Build history of the part. All positions in model axes, mm. Face numbers are marked on the shaded views. Round coordinates to 2 decimals unless told otherwise and drop trailing zeros. Loops run counter-clockwise (first coordinate to the right, second up) from the corner with the lowest first, then second, coordinate; pieces in that order, holes last. Notation, with made-up numbers: (-15, 78) - (-7, 78) arc R18 cw to (-7, 85) - close; hole circle Ø2 at (-2.75, 43.25). An arc over 180 degrees is marked (long way). Put each result on its own line as item: value. Start each with the question number.
from build123d import *

# Parameters (mm, degrees)
SKETCH051_R     = 40
PAD040_DEPTH    = 12
POCKET008_DEPTH = 12
FILLET002_R     = 1


with BuildPart() as part:
    # Sketch051 → Pad040 (new body)
    with BuildSketch(Plane.YZ.offset(67.95)):
        Circle(SKETCH051_R)
        with BuildLine():
            ThreePointArc((-1.4005, 2.125), (0, -2.545), (1.4005, 2.125))
            Line((-1.4005, 2.125), (1.4005, 2.125))
        make_face(mode=Mode.SUBTRACT)
    extrude(amount=PAD040_DEPTH)

    # Sketch052 (on Face5 of Pad040) → Pocket008 (cut)
    with BuildSketch(Plane.YZ.offset(79.95)):
        with BuildLine():
            ThreePointArc((-12.5, 31.618824), (-24.041631, 24.041631), (-31.618824, 12.5))
            ThreePointArc((-31.618824, 12.5), (-24.458371, -3.572618), (-7.720294, -8.99829))
            ThreePointArc((-12.5, 31.618824), (-22.685955, 9.830382), (-7.720294, -8.99829))
        make_face()
        with BuildLine():
            ThreePointArc((31.618824, 12.5), (24.041631, 24.041631), (12.5, 31.618824))
            ThreePointArc((12.5, 31.618824), (-3.572618, 24.458371), (-8.99829, 7.720294))
            ThreePointArc((31.618824, 12.5), (9.830382, 22.685955), (-8.99829, 7.720294))
        make_face()
        with BuildLine():
            ThreePointArc((12.5, -31.618824), (24.041631, -24.041631), (31.618824, -12.5))
            ThreePointArc((31.618824, -12.5), (24.458371, 3.572618), (7.720294, 8.99829))
            ThreePointArc((12.5, -31.618824), (22.685955, -9.830382), (7.720294, 8.99829))
        make_face()
        with BuildLine():
            ThreePointArc((-31.618824, -12.5), (-24.041631, -24.041631), (-12.5, -31.618824))
            ThreePointArc((-12.5, -31.618824), (3.572618, -24.458371), (8.99829, -7.720294))
            ThreePointArc((-31.618824, -12.5), (-9.830382, -22.685955), (8.99829, -7.720294))
        make_face()
    extrude(amount=-POCKET008_DEPTH, mode=Mode.SUBTRACT)

    # Fillet002
    fillet002_edges = [part.edges().sort_by_distance(p)[0] for p in [
        (67.95, 0, 2.125),
        (67.95, 0, -2.545),
        (67.95, -40, 0),
        (79.95, -40, 0),
        (79.95, 0, 2.125),
        (79.95, 0, -2.545),
    ]]
    fillet(fillet002_edges, radius=FILLET002_R)


solid = part.part
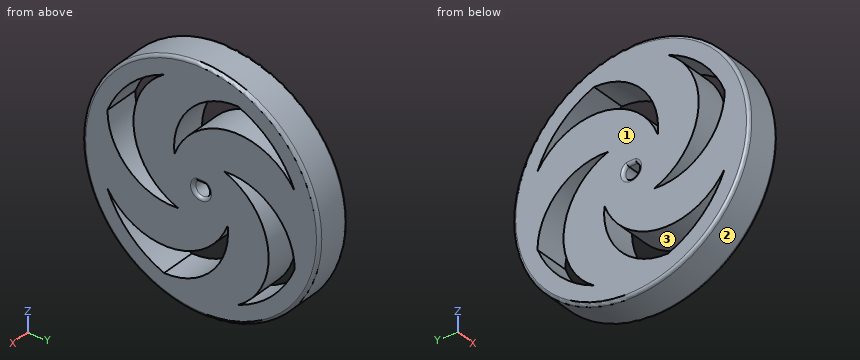
Item 1: Drill centre lines: probe 1 along Z at (x, y) = (73, 0) (3 decimals); probe 2 along Y at (x, z) = (72, -29); probe 3 along Y at (x, z) = (73.25, 26). Where is each one in solid material? Low to high. Write a range as [from, to].
Item 2: Drop flat-ended pins along their axis: pin 1 Ø1.4 at (x, y) = (72.5, 0) entering from -Z; pin 2 Ø6 at (y, z) = (0, 0) entering from +X; pin 3 Ø1 at (x, z) = (70, -10.5) entering from -Y. Give the stop position or say it passes through.
Item 3: Slice it at A-A (x = 72). Give the cut face in (y, z) (1 decimal), plus the area to 3 significant figures.
Item 4: Slice it at C-C (z = -19). Give the number of separate pieces and of enclosed holes in the cut face, plus the area to 3 significant figures.
Item 5: Slice it at B-B (y = 0). Give the cut face in (x, z) (3 decimals), plus the area to 3 significant figures.
Item 6: Two-plate mould, pull along Y, no slides. Class the marked faces 1, 2 and 3: pulls with the +Y half, pulls with the -Y half, needs draft (parallel to the pull), parting line crosses it, or undercut.
Computed values:
1. probe 1: z = [-40, -27.639], [-19.119, -2.545], [2.125, 19.119], [27.639, 40]
1. probe 2: y = [-27.55, -17.75], [-2.19, 15.8], [17.75, 27.55]
1. probe 3: y = [-30.4, -21.91], [-18.43, -2.04], [21.91, 30.4]
2. pin 1: stops at z = -40
2. pin 2: stops at x = 79.94
2. pin 3: stops at y = -38.73
3. outline: circle Ø80 at (0, 0); hole (-31.6, -12.5) arc R34 ccw to (-12.5, -31.6) arc R21.6 ccw to (9, -7.7) arc R22.8 cw to start; hole (-31.6, 12.5) arc R21.6 ccw to (-7.7, -9) arc R22.8 cw to (-12.5, 31.6) arc R34 ccw to start; hole (-9, 7.7) arc R22.8 cw to (31.6, 12.5) arc R34 ccw to (12.5, 31.6) arc R21.6 ccw to start; hole (-1.4, 2.1) arc R2.5 ccw (long way) to (1.4, 2.1) - close; hole (7.7, 9) arc R22.8 cw to (12.5, -31.6) arc R34 ccw to (31.6, -12.5) arc R21.6 ccw to start
3. area: 3,910 mm^2
4. separate pieces: 4
4. enclosed holes: 0
4. area: 648 mm^2
5. outline: (67.95, -39) arc R1 ccw to (68.95, -40) - (78.95, -40) arc R1 ccw to (79.95, -39) - (79.95, -27.639) - (67.95, -27.639) - close; (67.95, -19.119) - (79.95, -19.119) - (79.95, -3.545) arc R1 ccw to (78.95, -2.545) - (68.95, -2.545) arc R1 ccw to (67.95, -3.545) - close; (67.95, 3.125) arc R1 ccw to (68.95, 2.125) - (78.95, 2.125) arc R1 ccw to (79.95, 3.125) - (79.95, 19.119) - (67.95, 19.119) - close; (67.95, 27.639) - (79.95, 27.639) - (79.95, 39) arc R1 ccw to (78.95, 40) - (68.95, 40) arc R1 ccw to (67.95, 39) - close
5. area: 698 mm^2
6. face 1: needs draft
6. face 2: parting line crosses it
6. face 3: undercut
